Autodesk Inventor part; units mm, degrees
ref_plane "YZ Plane" through (0, 0, 0) normal (1, 0, 0) x (0, 1, 0)
ref_plane "XZ Plane" through (0, 0, 0) normal (0, 1, 0) x (-1, 0, 0)
ref_plane "XY Plane" through (0, 0, 0) normal (0, 0, 1) x (1, 0, 0)
sketch "草圖1" plane through (0, 0, 0) normal (0, 1, 0) x (-1, 0, 0)
  circle A0 centre (0, 0) radius 70
  circle A1 centre (0, 0) radius 25
  line L0 (-70, 10) -> (-10, 10)
  line L1 (-10, 10) -> (-10, -10)
  line L2 (-10, -10) -> (-70, -10)
  line L3 (-70, -10) -> (-70, 10)
  line L4 (0, 0) -> (0, -55)
  line L5 (0, 0) -> (35.3533, -42.1324)
  arc A2 (0, -55) -> (35.3533, -42.1324) centre (0, 0) ccw
  line L6 (0, 0) -> (51.6831, -18.8111)
  line L7 (0, 0) -> (51.6831, 18.8111)
  arc A3 (51.6831, -18.8111) -> (51.6831, 18.8111) centre (0, 0) ccw
  line L8 (0, 0) -> (35.3533, 42.1324)
  line L9 (0, 0) -> (0, 55)
  arc A4 (35.3533, 42.1324) -> (0, 55) centre (0, 0) ccw
  line L10 (-9.2, -7) -> (-36.8, -7)
  line L11 (-36.8, -7) -> (-36.8, -63)
  line L12 (-36.8, -63) -> (-9.2, -63)
  line L13 (-9.2, -63) -> (-9.2, -7)
  line L14 (-7.7, -14) -> (-10.7, -14)
  line L15 (-10.7, -14) -> (-10.7, -21)
  line L16 (-10.7, -21) -> (-7.7, -21)
  line L17 (-7.7, -21) -> (-7.7, -14)
  line L18 (-7.7, -49) -> (-10.7, -49)
  line L19 (-10.7, -49) -> (-10.7, -56)
  line L20 (-10.7, -56) -> (-7.7, -56)
  line L21 (-7.7, -56) -> (-7.7, -49)
  line L22 (-35.3, -14) -> (-38.3, -14)
  line L23 (-38.3, -14) -> (-38.3, -21)
  line L24 (-38.3, -21) -> (-35.3, -21)
  line L25 (-35.3, -21) -> (-35.3, -14)
  line L26 (-35.3, -42) -> (-38.3, -42)
  line L27 (-38.3, -42) -> (-38.3, -49)
  line L28 (-38.3, -49) -> (-35.3, -49)
  line L29 (-35.3, -49) -> (-35.3, -42)
  circle A5 centre (0, 0) radius 2
  line L30 (-1.5, 1.3229) -> (-1.5, -1.3229)
  point P0 (-23, -10)
  point P1 (-9.2, -14)
  point P2 (-9.2, -56)
  point P3 (-36.8, -14)
  point P4 (-36.8, -42)
  point P5 (16.0697, -19.1511)
  point P6 (0, -25)
  point P7 (-69.282, 10)
  point P8 (-69.282, -10)
  point P9 (16.0697, 19.1511)
  point P10 (0, 25)
  point P11 (23.4923, -8.5505)
  point P12 (23.4923, 8.5505)
  point P13 (-70, 0)
  point P14 (-10, 0)
  point P15 (-23, -7)
  dimension "d0" = 140
  dimension "d1" = 50
  dimension "d2" = 20
  dimension "d3" = 60
  dimension "d4" = 55
  dimension "d5" = 40
  dimension "d6" = 55
  dimension "d9" = 140
  dimension "d12" = 27.6
  dimension "d13" = 56
  dimension "d14" = 7
  dimension "d15" = 3
  dimension "d16" = 7
  dimension "d17" = 7
  dimension "d18" = 3
  dimension "d19" = 7
  dimension "d20" = 7
  dimension "d21" = 3
  dimension "d22" = 7
  dimension "d23" = 7
  dimension "d24" = 3
  dimension "d25" = 21
  dimension "d28" = 4
  dimension "d29" = 1.5
  dimension "d30" = 17
  dimension "d31" = 17
  dimension "d32" = 13
extrude "擠出1" add sketch "草圖1" along normal blind 3 contours A0 L12 L13 L20 L21 L18 A1 L4 A2 L5 L6 A3 L7 L8 A4 L9 L0 | A0 L11 L28 L29 L26 L24 L25 L22 L2 A1 L13 L18 L19 L20 L12 | A1 L9 A5 L4 L13 L16 L17 L14 L10 L1 L0 | A0 L2 L11 L22 L23 L24 L26 L27 L28 | A1 L8 A5 L9 | A1 L7 A5 L8 | A5 L8 L9 | L9 L4 A5 L30 | L2 L1 L10 L13 L14 L15 L16 A1 | A1 L6 A5 L7 | A5 L7 L8 | L5 A5 L4 | L6 A5 L5 | L7 A5 L6 | L30 A5 | A5 L5 A1 L4 | A5 L6 A1 L5
sketch "草圖2" plane through (0, 3, 0) normal (0, 1, 0) x (1, 0, 0)
  line L0 (-3, 13) -> (3, 13)
  line L1 (3, 13) -> (3, 10)
  line L2 (3, 10) -> (-3, 10)
  line L3 (-3, 10) -> (-3, 13)
  line L4 (-12.7583, 3.9019) -> (-9.7583, 9.0981)
  line L5 (-9.7583, 9.0981) -> (-7.1603, 7.5981)
  line L6 (-7.1603, 7.5981) -> (-10.1603, 2.4019)
  line L7 (-10.1603, 2.4019) -> (-12.7583, 3.9019)
  line L8 (-9.7583, -9.0981) -> (-12.7583, -3.9019)
  line L9 (-12.7583, -3.9019) -> (-10.1603, -2.4019)
  line L10 (-10.1603, -2.4019) -> (-7.1603, -7.5981)
  line L11 (-7.1603, -7.5981) -> (-9.7583, -9.0981)
  line L12 (3, -13) -> (-3, -13)
  line L13 (-3, -13) -> (-3, -10)
  line L14 (-3, -10) -> (3, -10)
  line L15 (3, -10) -> (3, -13)
  line L16 (-66, 3) -> (-63, 3)
  line L17 (-63, 3) -> (-63, -3)
  line L18 (-63, -3) -> (-66, -3)
  line L19 (-66, -3) -> (-66, 3)
  line L20 (-34.0981, -53.0596) -> (-28.9019, -56.0596)
  line L21 (-28.9019, -56.0596) -> (-30.4019, -58.6577)
  line L22 (-30.4019, -58.6577) -> (-35.5981, -55.6577)
  line L23 (-35.5981, -55.6577) -> (-34.0981, -53.0596)
  line L24 (28.9019, -56.0596) -> (34.0981, -53.0596)
  line L25 (34.0981, -53.0596) -> (35.5981, -55.6577)
  line L26 (35.5981, -55.6577) -> (30.4019, -58.6577)
  line L27 (30.4019, -58.6577) -> (28.9019, -56.0596)
  line L28 (63, -3) -> (63, 3)
  line L29 (63, 3) -> (66, 3)
  line L30 (66, 3) -> (66, -3)
  line L31 (66, -3) -> (63, -3)
  line L32 (34.0981, 53.0596) -> (28.9019, 56.0596)
  line L33 (28.9019, 56.0596) -> (30.4019, 58.6577)
  line L34 (30.4019, 58.6577) -> (35.5981, 55.6577)
  line L35 (35.5981, 55.6577) -> (34.0981, 53.0596)
  line L36 (-28.9019, 56.0596) -> (-34.0981, 53.0596)
  line L37 (-34.0981, 53.0596) -> (-35.5981, 55.6577)
  line L38 (-35.5981, 55.6577) -> (-30.4019, 58.6577)
  line L39 (-30.4019, 58.6577) -> (-28.9019, 56.0596)
  point P0 (0, 0)
  point P1 (0, 10)
  point P2 (-8.6603, 5)
  point P3 (-8.6603, -5)
  point P4 (0, -10)
  point P5 (-63, 0)
  point P6 (-31.5, -54.5596)
  point P7 (31.5, -54.5596)
  point P8 (63, 0)
  point P9 (31.5, 54.5596)
  point P10 (-31.5, 54.5596)
  dimension "d33" = 3
  dimension "d34" = 6
  dimension "d35" = 10
  dimension "d38" = 180
  dimension "d49" = 3
  dimension "d50" = 6
  dimension "d51" = 63
  dimension "d54" = 360
extrude "擠出2" cut sketch "草圖2" against normal through all contours L0 L1 L2 L3 | L4 L5 L6 L7 | L8 L9 L10 L11 | L12 L13 L14 L15 | L16 L17 L18 L19 | L20 L21 L22 L23 | L24 L25 L26 L27 | L32 L33 L34 L35 | L36 L37 L38 L39
properties part number "rolling_plate_top"
Part model, mm, in its own coordinate system. A direction names the side the tool comes from. Coordinates: 2 decimals unless noted, no trailing zeros. Loops run counter-clockwise (first coordinate to the right, second up) from the corner with the lowest first, then second, coordinate; pieces in that order, holes last. Notation, with made-up numbers: M 67.5,-10.5 L 114.5,-10.5 A32 ccw 114.5,15.5 Z; hole C -28,31 d9. An arc over 180 degrees is marked long. Use a Markdown table: item, result. Add a question column.
Q1. Which spindle directions (+Z, -Z, +X, -X, +Y, -Y) get a long thin tool onto all of the face, cutting with end or side? Do faces 1 (the flat face through (40, 1, 10)), 2 (the cylindrical face through (-18.558, 1.479, 51.774)). Say none if no direction does.
Q2. Pin check, flat tips, straight feed: P1, Ø0.9, axis at x = 43, y = 1.5, coming from the +Z side; P2, Ø1.5, axis at x = 48, y = 2, coming from the -Z side; P3, Ø0.9, axis at y = 2, z = -1, coming from the -X side. Stop position of each tip, or through.
Q3. Mould opens along Z. For faces 3 (the flat face through (33.036, 1.521, 57.137)), 4 (the flat face through (1, 3, 1)) say: +Z half, -Z half, draft (parallel to the pull), parting line (faces both ways), or undercut.
Q4. Cut at D-D (y = 1.3). Give the number of separate pieces and of enclosed holes in the cut face, and give its area (3 significant figures).
Q5. Cut at C-C (z = -27). Write the cut outline in (x, y), and give its area (3 significant figures).
Q6. Probe L1, parallel to Z at x = 2, y = 2.25; L2, parallel to Z at x = -29, y = 1.15; L3, parallel to X at y = 0.9, z = -43.5. List the from-to ranges inside material, lowest first.
Q7. Cut at A-A (z = 0). Write the cut outline in (x, y), and give its area (3 significant figures).
Q8. Cut at B-B (x = -49). Write the cut outline in (y, z), and give its area (3 significant figures).
Worked out:
| question | item | result |
|---|---|---|
| 1 | face 1 | +X, +Y, -Y |
| 1 | face 2 | +Y, -Y |
| 2 | P1 | stops at z = 55.58 |
| 2 | P2 | stops at z = -51.65 |
| 2 | P3 | stops at x = -70 |
| 3 | face 3 | undercut |
| 3 | face 4 | draft |
| 4 | separate pieces | 1 |
| 4 | enclosed holes | 16 |
| 4 | area | 11,400 mm2 |
| 5 | outline | M -64.58,0 L -22.66,0 L -22.66,3 L -64.58,3 Z; M 0,0 L 64.58,0 L 64.58,3 L 0,3 Z |
| 5 | area | 320 mm2 |
| 6 | L1 | z = -69.97 to -13, -10 to 10, 13 to 69.97 |
| 6 | L2 | z = -63.71 to -56.23, -56 to -46.73, -34.56 to -10.56, 10.56 to 34.56, 46.73 to 56, 56.23 to 63.71 |
| 6 | L3 | x = -54.84 to -33.66, 0 to 35.3, 38.3 to 54.84 |
| 7 | outline | M -70,0 L -66,0 L -66,3 L -70,3 Z; M -63,0 L -55,0 L -55,3 L -63,3 Z; M -25,0 L 10,0 L 10,3 L -25,3 Z |
| 7 | area | 141 mm2 |
| 8 | outline | M 0,-49.99 L 3,-49.99 L 3,-17.83 L 0,-17.83 Z; M 0,17.83 L 3,17.83 L 3,49.99 L 0,49.99 Z |
| 8 | area | 193 mm2 |
